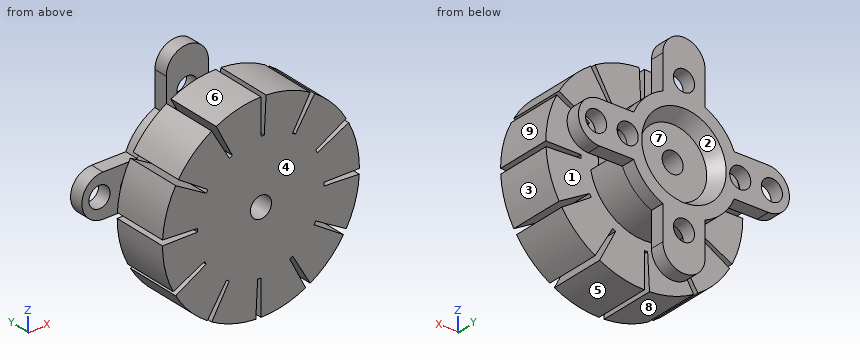
from build123d import *

# Parameters (mm, degrees)
SKETCH1_W           = 6
SKETCH1_H           = 6
BOSS_EXTRUDE1_DEPTH = 2
SKETCH2_R           = 1.5
CUT_EXTRUDE1_DEPTH  = 3
SKETCH3_R           = 6
CUT_EXTRUDE2_DEPTH  = 3
CUT_EXTRUDE2_TAPER  = 30
BOSS_EXTRUDE2_DEPTH = 13
SKETCH5_R           = 14
BOSS_EXTRUDE3_DEPTH = 8
SKETCH6_R           = 1.5
CUT_EXTRUDE3_DEPTH  = 14
CUT_EXTRUDE5_DEPTH  = 8
CIRPATTERN1_COUNT   = 12


with BuildPart() as part:
    # Sketch1 → Boss-Extrude1 (new body)
    with BuildSketch(Plane(origin=(0, 0, 0), x_dir=(1, 0, 0), z_dir=(0, 1, 0))):
        with BuildLine():
            Line((-12, -3), (-7.145802964, -3))
            ThreePointArc((-7.145802964, -3), (-7.75, 0), (-7.145802964, 3))
            Line((-7.145802964, 3), (-12, 3))
            ThreePointArc((-12, 3), (-15, 0), (-12, -3))
        make_face()
        with BuildLine():
            Line((-7.145802964, -3), (-3, -3))
            Line((-3, -3), (-3, 3))
            Line((-3, 3), (-7.145802964, 3))
            ThreePointArc((-7.145802964, 3), (-7.75, 0), (-7.145802964, -3))
        make_face()
        with BuildLine():
            Line((3, -3), (3, -7.145802964))
            ThreePointArc((3, -7.145802964), (5.480077554, -5.480077554), (7.145802964, -3))
            Line((7.145802964, -3), (3, -3))
        make_face()
        with BuildLine():
            Line((-3, -3), (-3, -7.145802964))
            ThreePointArc((-3, -7.145802964), (0, -7.75), (3, -7.145802964))
            Line((3, -7.145802964), (3, -3))
            Line((3, -3), (-3, -3))
        make_face()
        with BuildLine():
            ThreePointArc((-7.145802964, -3), (-5.480077554, -5.480077554), (-3, -7.145802964))
            Line((-3, -7.145802964), (-3, -3))
            Line((-3, -3), (-7.145802964, -3))
        make_face()
        with BuildLine():
            Line((-7.145802964, 3), (-3, 3))
            Line((-3, 3), (-3, 7.145802964))
            ThreePointArc((-3, 7.145802964), (-5.480077554, 5.480077554), (-7.145802964, 3))
        make_face()
        with BuildLine():
            Line((-3, 7.145802964), (-3, 3))
            Line((-3, 3), (3, 3))
            Line((3, 3), (3, 7.145802964))
            ThreePointArc((3, 7.145802964), (0, 7.75), (-3, 7.145802964))
        make_face()
        with BuildLine():
            Line((-3, 12), (-3, 7.145802964))
            ThreePointArc((-3, 7.145802964), (0, 7.75), (3, 7.145802964))
            Line((3, 7.145802964), (3, 12))
            ThreePointArc((3, 12), (0, 15), (-3, 12))
        make_face()
        Rectangle(SKETCH1_W, SKETCH1_H)
        with BuildLine():
            Line((3, 3), (3, -3))
            Line((3, -3), (7.145802964, -3))
            ThreePointArc((7.145802964, -3), (7.597449341, -1.530118791), (7.75, 0))
            ThreePointArc((7.75, 0), (7.597449341, 1.530118791), (7.145802964, 3))
            Line((7.145802964, 3), (3, 3))
        make_face()
        with BuildLine():
            Line((3, 7.145802964), (3, 3))
            Line((3, 3), (7.145802964, 3))
            ThreePointArc((7.145802964, 3), (5.480077554, 5.480077554), (3, 7.145802964))
        make_face()
        with BuildLine():
            ThreePointArc((7.75, 0), (7.597449341, -1.530118791), (7.145802964, -3))
            Line((7.145802964, -3), (12, -3))
            ThreePointArc((12, -3), (15, 0), (12, 3))
            Line((12, 3), (7.145802964, 3))
            ThreePointArc((7.145802964, 3), (7.597449341, 1.530118791), (7.75, 0))
        make_face()
        with BuildLine():
            Line((-3, -7.145802964), (-3, -12))
            ThreePointArc((-3, -12), (0, -15), (3, -12))
            Line((3, -12), (3, -7.145802964))
            ThreePointArc((3, -7.145802964), (0, -7.75), (-3, -7.145802964))
        make_face()
    extrude(amount=BOSS_EXTRUDE1_DEPTH)

    # Sketch2 → Cut-Extrude1 (cut, through all)
    with BuildSketch(Plane(origin=(0, 2, 0), x_dir=(1, 0, 0), z_dir=(0, 1, 0))):
        with Locations((8, 0)):
            Circle(SKETCH2_R)
        with Locations((12.5, 0)):
            Circle(SKETCH2_R)
        with Locations((0, 9.5)):
            Circle(SKETCH2_R)
        with Locations((0, -9.5)):
            Circle(SKETCH2_R)
        with Locations((-12.5, 0)):
            Circle(SKETCH2_R)
        with Locations((-8, 0)):
            Circle(SKETCH2_R)
    extrude(amount=-CUT_EXTRUDE1_DEPTH, mode=Mode.SUBTRACT)

    # Sketch3 → Cut-Extrude2 (cut, through all)
    with BuildSketch(Plane(origin=(0, 2, 0), x_dir=(1, 0, 0), z_dir=(0, 1, 0))):
        Circle(SKETCH3_R)
    extrude(amount=-CUT_EXTRUDE2_DEPTH, taper=CUT_EXTRUDE2_TAPER, mode=Mode.SUBTRACT)

    # Sketch4 → Boss-Extrude2 (add)
    with BuildSketch(Plane.XZ):
        with BuildLine():
            ThreePointArc((-7.61328125, -1.449292451), (0, -7.75), (7.61328125, -1.449292451))
            ThreePointArc((7.61328125, -1.449292451), (6.5, 0), (7.61328125, 1.449292451))
            ThreePointArc((7.61328125, 1.449292451), (0, 7.75), (-7.61328125, 1.449292451))
            ThreePointArc((-7.61328125, 1.449292451), (-6.5, 0), (-7.61328125, -1.449292451))
        make_face()
    extrude(amount=BOSS_EXTRUDE2_DEPTH)

    # Sketch5 → Boss-Extrude3 (add)
    with BuildSketch(Plane.XZ.offset(13)):
        Circle(SKETCH5_R)
    extrude(amount=-BOSS_EXTRUDE3_DEPTH)

    # Sketch6 → Cut-Extrude3 (cut, through all)
    with BuildSketch(Plane(origin=(0, 0, 0), x_dir=(1, 0, 0), z_dir=(0, 1, 0))):
        Circle(SKETCH6_R)
    extrude(amount=-CUT_EXTRUDE3_DEPTH, mode=Mode.SUBTRACT)

    # Sketch7 → Cut-Extrude5 (cut)
    with BuildSketch(Plane.XZ.offset(13)):
        with BuildLine():
            Line((14, 0), (9, 0))
            ThreePointArc((9, 0), (8.996915925, -0.235592535), (8.987665813, -0.471023606))
            Line((8.987665813, -0.471023606), (13.980813487, -0.732703387))
            ThreePointArc((13.980813487, -0.732703387), (13.99520255, -0.366477276), (14, 0))
        make_face()
    cut_extrude5 = extrude(amount=-CUT_EXTRUDE5_DEPTH, mode=Mode.SUBTRACT)

    # CirPattern1: Cut-Extrude5 ×12 about axis
    cirpattern1_axis = Axis((0, -13, 0), (0, -1, 0))
    for i in range(1, CIRPATTERN1_COUNT):
        add(cut_extrude5.rotate(cirpattern1_axis, i * 360 / CIRPATTERN1_COUNT), mode=Mode.SUBTRACT)


solid = part.part
For this review, take the finished solid that the model builds, in its own axes (mm). Face numbers are marked on the shaded views. A direction names the side the tool comes from. Round coordinates to 2 decimals unless told otherwise and drop trailing zeros. Loops run counter-clockwise (first coordinate to the right, second up) from the corner with the lowest first, then second, coordinate; pieces in that order, holes last. Notation, with made-up numbers: (78.5, 79) - (106.5, 79) arc R24 cw to (106.5, 106) - close; hole circle Ø9 at (78, 72). An arc over 180 degrees is marked (long way). Use one line per item in the form item = value.
Item 1: Tool access review of the marked faces 5, 6, 7, 8 and 9: name each direction out of +Z, -Z, +X, -X, +Y, -Y from which nothing blocks a thin tool from reaching the whole face with its end or side.
Answers:
face_5 = -Z, +X, -Y
face_6 = +Z, -X, -Y
face_7 = +Y
face_8 = -Z, -X, -Y
face_9 = +Z, +X, -Y
Item 2: Clearance check with flat-ended pins moving along their axes: P1, Ø4, axis at x = -8.5, y = -2, coming from the -Z side; P2, Ø1, axis at y = 1, z = -9, coming from the +X side; P3, Ø1.5, axis at x = 1.5, y = -4, coming from the -Z side; P4, Ø10.5, axis at x = -0.5, z = -1, coming from the +Y side. State where each tip first meets the part, or that it passes through.
Answers:
P1 = -4.22
P2 = 3
P3 = -7.71
P4 = 2
Item 3: For line 1 (X direction, y = 1.6, z = 0); line 2 (Z direction, x = 0, y = 1.25); line 3 (X direction, y = 1, z = 1), list the stretches that pass through material, from the lowest coordinate up.
Answers:
line_1 = -15 to -14, -11 to -9.5, -6.5 to -5.77, 5.77 to 6.5, 9.5 to 11, 14 to 15
line_2 = -15 to -11, -8 to -5.57, 5.57 to 8, 11 to 15
line_3 = -14.83 to -13.62, -11.38 to -9.12, -6.88 to -5.33, 5.33 to 6.88, 9.12 to 11.38, 13.62 to 14.83
Item 4: Mouldability with a two-part tool opening along Y and no side actions: class the marked faces 1, 2, 3 and 4 as +Y half, -Y half, draft (parallel to the pull), parting line (faces both ways), or undercut.
Answers:
face_1 = undercut
face_2 = +Y half
face_3 = draft
face_4 = -Y half
Item 5: Consider section A-A on z = -9.5. Write out the cut boundary in (x, y).
Answers:
outline = (-10.28, -13) - (-6.17, -13) - (-6.17, -5) - (-10.28, -5) - close; (-5.48, -13) - (-0.5, -13) - (-0.5, -5) - (-5.48, -5) - close; (-3, 0) - (-1.5, 0) - (-1.5, 2) - (-3, 2) - close; (0, -13) - (4.84, -13) - (4.84, -5) - (0, -5) - close; (1.5, 0) - (3, 0) - (3, 2) - (1.5, 2) - close; (5.48, -13) - (10.28, -13) - (10.28, -5) - (5.48, -5) - close
